Design review of the part shown in the three views and the two pictorial views. Dimensions are in mm from the part's minimum x, y and z. A direction names the side the tool comes from. Coordinates: 2 decimals unless noted, no trailing zeros. Loops run counter-clockwise (first coordinate to the right, second up) from the corner with the lowest first, then second, coordinate; pieces in that order, holes last. Notation, with made-up numbers: (85, -6) -> (141, -6) arc R18 cw to (141, 0) -> close; hole circle Ø5 at (-33, 6). An arc over 180 degrees is marked (long way). One line per item, written item: value. Start each with the question number.
1. Draft analysis for pull direction X (two halves, no side actions). For the marked faces 3, 4 and 5, state which applies: pulls with the +X half, pulls with the -X half, needs draft (parallel to the pull), parting line crosses it, or undercut.
2. For probe 1 along X at (y, z) = (71, 12.75); probe 2 along X at (y, z) = (95.5, 1); probe 3 along Y at (x, z) = (4.5, 19), list the stretches that pass through material, from the lowest coordinate up.
3. Insertion check: pin 1 (8 mm diameter, centred on x = 31, y = 31, fed in from +Z). The pin has a flat end and moves straight along its axis. Give the tip position at first contact, or say it passes through.
4. Machinability: for the marked faces 1 and 2, which of the approach directions +Z, -Z, +X, -X, +Y, -Y give a long, thin tool a straight path to every point of the face, cutting with its end or side? Answer none if there is none.
5. Add section D-D on x = 32.5. Write out the cut boundary in (y, z).
6. Add section B-B on x = 23.5. Write out the cut boundary in (y, z) (1 decimal), plus the area to 3 significant figures.
7. Add section A-A on z = 2. Write out the cut boundary in (x, y) (1 decimal), plus the area to 3 significant figures.
8. Add section C-C on y = 67.5. Write out the cut boundary in (x, z).
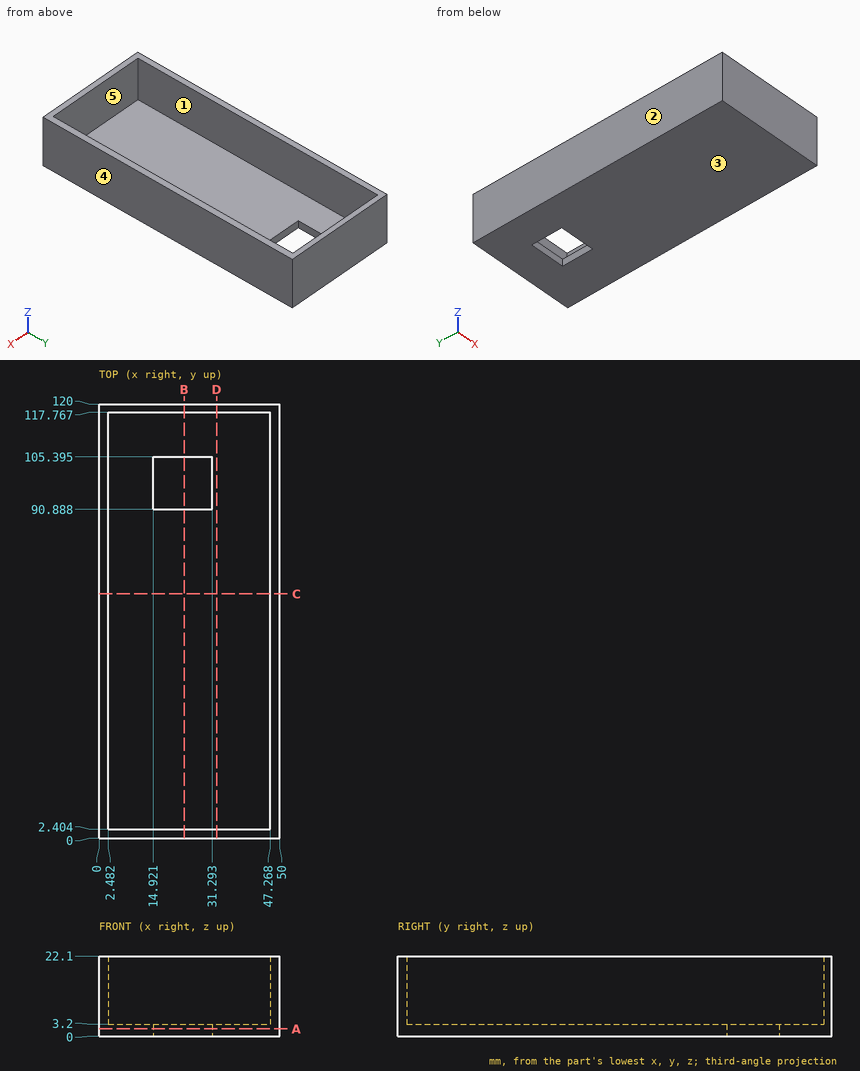
Worked answers:
1. face 3: needs draft
1. face 4: pulls with the +X half
1. face 5: undercut
2. probe 1: x = 0 to 2.48, 47.27 to 50
2. probe 2: x = 0 to 14.92, 31.29 to 50
2. probe 3: y = 0 to 2.4, 117.77 to 120
3. pin 1: stops at z = 3.2
4. face 1: +Z
4. face 2: +Z, -Z, -X, +Y, -Y
5. outline: (0, 0) -> (120, 0) -> (120, 22.1) -> (117.77, 22.1) -> (117.77, 3.2) -> (2.4, 3.2) -> (2.4, 22.1) -> (0, 22.1) -> close
6. outline: (0, 0) -> (90.9, 0) -> (90.9, 3.2) -> (2.4, 3.2) -> (2.4, 22.1) -> (0, 22.1) -> close; (105.4, 0) -> (120, 0) -> (120, 22.1) -> (117.8, 22.1) -> (117.8, 3.2) -> (105.4, 3.2) -> close
6. area: 425 mm²
7. outline: (0, 0) -> (50, 0) -> (50, 120) -> (0, 120) -> close; hole (14.9, 90.9) -> (31.3, 90.9) -> (31.3, 105.4) -> (14.9, 105.4) -> close
7. area: 5,760 mm²
8. outline: (0, 0) -> (50, 0) -> (50, 22.1) -> (47.27, 22.1) -> (47.27, 3.2) -> (2.48, 3.2) -> (2.48, 22.1) -> (0, 22.1) -> close
